Part model, mm, in its own coordinate system. A direction names the side the tool comes from. Give positions to 0.01 mm unless a question says otherwise; leave off trailing zeros. Loops run counter-clockwise (first coordinate to the right, second up) from the corner with the lowest first, then second, coordinate; pieces in that order, holes last. Notation, with made-up numbers: M 88,53.5 L 96,53.5 A25 cw 96,81.5 Z; hole C 83,-35.5 d2. An arc over 180 degrees is marked long. Put each result on its own line as item: value. Start each with the question number.
```python
from build123d import *

# Parameters (mm, degrees)
CROQUIS1_W              = 14.4
CROQUIS1_H              = 14.4
SALIENTE_EXTRUIR1_DEPTH = 2
CROQUIS2_W              = 1.894290675
CROQUIS2_H              = 1
SALIENTE_EXTRUIR2_DEPTH = 4


with BuildPart() as part:
    # Croquis1 → Saliente-Extruir1 (new body)
    with BuildSketch(Plane.XY):
        Rectangle(CROQUIS1_W, CROQUIS1_H)
    extrude(amount=SALIENTE_EXTRUIR1_DEPTH)

    # Croquis2 → Saliente-Extruir2 (add)
    with BuildSketch(Plane.XY.offset(2)):
        with Locations((-2.082854662, -6.7)):
            Rectangle(CROQUIS2_W, CROQUIS2_H)
        with Locations((-6.252854663, -6.7)):
            Rectangle(CROQUIS2_W, CROQUIS2_H)
        with Locations((2.087145337, -6.7)):
            Rectangle(CROQUIS2_W, CROQUIS2_H)
        with Locations((6.257145338, -6.7)):
            Rectangle(CROQUIS2_W, CROQUIS2_H)
        with Locations((-2.082854662, -4.47)):
            Rectangle(CROQUIS2_W, CROQUIS2_H)
        with Locations((2.087145337, -4.47)):
            Rectangle(CROQUIS2_W, CROQUIS2_H)
        with Locations((6.257145338, -4.47)):
            Rectangle(CROQUIS2_W, CROQUIS2_H)
        with Locations((-2.082854662, -2.24)):
            Rectangle(CROQUIS2_W, CROQUIS2_H)
        with Locations((2.087145337, -2.24)):
            Rectangle(CROQUIS2_W, CROQUIS2_H)
        with Locations((6.257145338, -2.24)):
            Rectangle(CROQUIS2_W, CROQUIS2_H)
        with Locations((-2.082854662, -0.01)):
            Rectangle(CROQUIS2_W, CROQUIS2_H)
        with Locations((2.087145337, -0.01)):
            Rectangle(CROQUIS2_W, CROQUIS2_H)
        with Locations((6.257145338, -0.01)):
            Rectangle(CROQUIS2_W, CROQUIS2_H)
        with Locations((-2.082854662, 2.22)):
            Rectangle(CROQUIS2_W, CROQUIS2_H)
        with Locations((2.087145337, 2.22)):
            Rectangle(CROQUIS2_W, CROQUIS2_H)
        with Locations((6.257145338, 2.22)):
            Rectangle(CROQUIS2_W, CROQUIS2_H)
        with Locations((-2.082854662, 4.45)):
            Rectangle(CROQUIS2_W, CROQUIS2_H)
        with Locations((2.087145337, 4.45)):
            Rectangle(CROQUIS2_W, CROQUIS2_H)
        with Locations((6.257145338, 4.45)):
            Rectangle(CROQUIS2_W, CROQUIS2_H)
        with Locations((-2.082854662, 6.68)):
            Rectangle(CROQUIS2_W, CROQUIS2_H)
        with Locations((2.087145337, 6.68)):
            Rectangle(CROQUIS2_W, CROQUIS2_H)
        with Locations((6.257145338, 6.68)):
            Rectangle(CROQUIS2_W, CROQUIS2_H)
        with Locations((-6.252854663, -4.47)):
            Rectangle(CROQUIS2_W, CROQUIS2_H)
        with Locations((-6.252854663, -2.24)):
            Rectangle(CROQUIS2_W, CROQUIS2_H)
        with Locations((-6.252854663, -0.01)):
            Rectangle(CROQUIS2_W, CROQUIS2_H)
        with Locations((-6.252854663, 2.22)):
            Rectangle(CROQUIS2_W, CROQUIS2_H)
        with Locations((-6.252854663, 4.45)):
            Rectangle(CROQUIS2_W, CROQUIS2_H)
        with Locations((-6.252854663, 6.68)):
            Rectangle(CROQUIS2_W, CROQUIS2_H)
    extrude(amount=SALIENTE_EXTRUIR2_DEPTH)


solid = part.part
```
1) Band-saw the part on C-C on z = 2.55. State how many separate pieces and enclosed holes the cut face has, then the cut area to 3 significant figures.
2) Band-saw the part on D-D on y = -6. Give the cut face in (x, z), then the cut area to 3 significant figures.
3) Wall check: L1, parallel to X at y = 4.25, z = 5.35; L2, parallel to Z at x = 3.5, y = 5.5; L3, parallel to X at y = -2, z = 1. Give the ranges that are in metal, low to high.
4) Pin check, flat tips, straight feed: pin 1 Ø1.5 at (x, z) = (2, 5) entering from +Y; pin 2 Ø6 at (x, y) = (5, -3.5) entering from -Z. Stop position of each tip, or through.
5) Which spindle directions (+Z, -Z, +X, -X, +Y, -Y) get a long thin tool onto all of the face, cutting with end or side? Do faces 1 (the flat face through (-6.3, -4.5, 6)), 2 (the flat face through (-6, 7.18, 4)), 3 (the flat face through (-5.306, -4.5, 4)), 4 (the flat face through (2, -3.97, 4)). Say none if no direction does.
6) Mould opens along X. For faces 5 (the flat face through (2, 7, 6)), 6 (the flat face through (1.14, 2, 4)) say: +X half, -X half, draft (parallel to the pull), parting line (faces both ways), or undercut.
Evaluation:
1. separate pieces: 28
1. enclosed holes: 0
1. area: 53.0 mm2
2. outline: M -7.2,0 L 7.2,0 L 7.2,2 L -7.2,2 Z
2. area: 28.8 mm2
3. L1: -7.2 to -5.31, -3.03 to -1.14, 1.14 to 3.03, 5.31 to 7.2
3. L2: 0 to 2
3. L3: -7.2 to 7.2
4. pin 1: y = 7.18
4. pin 2: z = 0
5. face 1: +Z, +X, -X, +Y, -Y
5. face 2: +Z, +X, -X, +Y
5. face 3: +Z, +Y, -Y
5. face 4: +Z, +X, -X
6. face 5: draft
6. face 6: undercut
